Check sheet for the modelled part. Datum: model origin and axes. Units: mm. A direction names the side the tool comes from. Round coordinates to 2 decimals unless told otherwise and drop trailing zeros. Order: outer loops, then holes, each group sorted by start corner. A loop starts at its lowest first (then second) coordinate and runs counter-clockwise, first axis right, second up.
(1) Sectioned sample at B-B, the plane y = -4. Enter the section's corners in (x, z).
(2) Thickness scan on probe 1 along Y at (x, z) = (-9.75, 39); probe 2 along X at (y, z) = (-11.75, 120.65). Record the ranges inside material, lowest first.
(3) Mould release check, pull along Z, two halves, no side actions. Record for faces 3 (the flat face through (-11.3, 0.1, 260.35)), 4 (the flat face through (0, 12.7, 128)), 5 (the cylindrical face through (-0.43, 11.917, 122.587)): released by +Z, released by -Z, zero draft, split by the parting line, or undercut.
(4) Tool access check on faces 1 (the flat face through (0, -11.112, 128)), 2 (the cylindrical face through (-0.43, -11.895, 224.187)). Record the directions out of +Z, -Z, +X, -X, +Y, -Y that give a thin tool (end or side, any length) a straight path to the whole face; none if there is none.
(5) Sectioned sample at A-A, the plane z = 75. Enter the section's corners in (x, y).
```python
from build123d import *

# Parameters (mm, degrees)
SKETCH1_W           = 25.4
SKETCH1_H           = 25.4
SKETCH1_W_2         = 22.225
SKETCH1_H_2         = 22.225
BOSS_EXTRUDE1_DEPTH = 260.35
SKETCH2_R           = 1.984375
SKETCH2_R_2         = 3.175
CUT_EXTRUDE1_DEPTH  = 26.4


with BuildPart() as part:
    # Sketch1 → Boss-Extrude1 (new body)
    with BuildSketch(Plane.XY):
        Rectangle(SKETCH1_W, SKETCH1_H)
        Rectangle(SKETCH1_W_2, SKETCH1_H_2, mode=Mode.SUBTRACT)
    extrude(amount=BOSS_EXTRUDE1_DEPTH)

    # Sketch2 → Cut-Extrude1 (cut, through all)
    with BuildSketch(Plane(origin=(0, 12.7, 0), x_dir=(1, 0, 0), z_dir=(0, 1, 0))):
        with Locations((0, -247.65)):
            Circle(SKETCH2_R)
        with Locations((0, -222.25)):
            Circle(SKETCH2_R)
        with Locations((0, -196.85)):
            Circle(SKETCH2_R)
        with Locations((0, -171.45)):
            Circle(SKETCH2_R)
        with Locations((0, -146.05)):
            Circle(SKETCH2_R)
        with Locations((0, -120.65)):
            Circle(SKETCH2_R)
        with Locations((0, -95.25)):
            Circle(SKETCH2_R)
        with Locations((0, -69.85)):
            Circle(SKETCH2_R)
        with Locations((0, -44.45)):
            Circle(SKETCH2_R)
        with Locations((0, 6.35)):
            Circle(SKETCH2_R)
        with Locations((0, 31.75)):
            Circle(SKETCH2_R)
        with Locations((0, -19.05)):
            Circle(SKETCH2_R_2)
    extrude(amount=-CUT_EXTRUDE1_DEPTH, mode=Mode.SUBTRACT)


solid = part.part
```
Derived:
1. outline: (-12.7, 0) - (-11.11, 0) - (-11.11, 260.35) - (-12.7, 260.35) - close; (11.11, 0) - (12.7, 0) - (12.7, 260.35) - (11.11, 260.35) - close
2. probe 1: y = -12.7 to -11.11, 11.11 to 12.7
2. probe 2: x = -12.7 to -1.98, 1.98 to 12.7
3. face 3: released by +Z
3. face 4: zero draft
3. face 5: undercut
4. face 1: +Z, -Z
4. face 2: +Y, -Y
5. outline: (-12.7, -12.7) - (12.7, -12.7) - (12.7, 12.7) - (-12.7, 12.7) - close; hole (-11.11, -11.11) - (11.11, -11.11) - (11.11, 11.11) - (-11.11, 11.11) - close
